Could you check a few things on this model? Use its own coordinates, in mm. A direction names the side the tool comes from. Give positions to 0.01 mm unless a question says otherwise; leave off trailing zeros. Order: outer loops, then holes, each group sorted by start corner. A loop starts at its lowest first (then second) coordinate and runs counter-clockwise, first axis right, second up. Notation, with made-up numbers: (71.5, 86.25) - (93.5, 86.25) arc R36 ccw to (93.5, 120.25) - close; hole circle Ø4 at (31.25, -6). An arc over 180 degrees is marked (long way). One line per question, with ' | ' between items. Start each with the question number.
1. Imagine slicing it at C-C (y = -45). Please give me the cut outline in (x, z), and give its area (3 significant figures).
2. If we mould it in two halves opening along Y, with no side actions, what happens to faces 1 (the cylindrical face through (-0.2, 18.95, -0.22)), 2 (the flat face through (-3, -54.33, 2)), 3 (the cylindrical face through (-3.905, -56.056, 0.867))? For each: released by +Y, released by -Y, zero draft, split by the parting line, or undercut.
3. I need wall thicknesses on probe 1 along X at (y, z) = (-36.5, -5.5); probe 2 along X at (y, z) = (3, 8). Which ranges of each line are inside material? Lowest first, please. Write a range as from..to.
4. For P1, Ø6.5, axis at x = 0.5, z = 1, coming from the +Y side; P2, Ø8, axis at x = 4.5, y = -24.5, coming from the -Z side; P3, Ø12, axis at x = 11.5, z = -13, coming from the -Y side, each with a flat end and sliding along its axis, tell me the tip position at first contact or that it passes through.
5. Which directions (+Z, -Z, +X, -X, +Y, -Y) give clear straight access to the entire face, cutting with the end or side of a thin tool? Please do faces 4 (the flat face through (0, -57.07, 0)), 5 (the cylindrical face through (-1.93, -54.71, 2.52)), 6 (the flat face through (-4.1, -39.57, -1.3)).
6. Imagine slicing it at D-D (y = -7.5). Please give me the cut outline in (x, z), and give its area (3 significant figures).
7. Imagine slicing it at A-A (z = 0). Please give me the cut outline in (x, y) (3 decimals).
8. Imagine slicing it at B-B (x = 0). Please give me the cut outline in (y, z) (3 decimals).
```python
from build123d import *

# Parameters (mm, degrees)
SKETCH1_R               = 16
BOSS_EXTRUDE1_DEPTH     = 24
SKETCH2_R               = 6.35
BOSS_EXTRUDE2_DEPTH     = 39.57
SKETCH3_R               = 4
BOSS_EXTRUDE3_DEPTH     = 17.5
CUT_EXTRUDE1_DEPTH      = 62.392058933
CUT_EXTRUDE1_DEPTH_BACK = 62.392058933
SKETCH4_R               = 19.05
CUT_EXTRUDE2_START      = -2
SKETCH5_R               = 4.571040919
SKETCH5_R_2             = 3.175
CUT_EXTRUDE2_DEPTH      = 0.74


with BuildPart() as part:
    # Sketch1 → Boss-Extrude1 (new body)
    with BuildSketch(Plane(origin=(0, 0, 0), x_dir=(1, 0, 0), z_dir=(0, 1, 0))):
        with Locations(Location((0, 0, 0), (0, 0, 270))):
            Circle(SKETCH1_R)
    extrude(amount=BOSS_EXTRUDE1_DEPTH)

    # Sketch2 → Boss-Extrude2 (add)
    with BuildSketch(Plane.XZ):
        with Locations(Location((0, 0, 0), (0, 0, 270))):
            Circle(SKETCH2_R)
    extrude(amount=BOSS_EXTRUDE2_DEPTH)

    # Sketch3 → Boss-Extrude3 (add)
    with BuildSketch(Plane.XZ.offset(39.57)):
        with Locations(Location((0, 0, 0), (0, 0, 270))):
            Circle(SKETCH3_R)
    extrude(amount=BOSS_EXTRUDE3_DEPTH)

    # Sketch4 → Cut-Extrude1 (cut, two sides: drawn at the far end of the back side and taken through both)
    with BuildSketch(Plane.XY.offset(-CUT_EXTRUDE1_DEPTH_BACK)):
        with Locations((0, 38)):
            Circle(SKETCH4_R)
    extrude(amount=CUT_EXTRUDE1_DEPTH + CUT_EXTRUDE1_DEPTH_BACK, mode=Mode.SUBTRACT)

    # Sketch5 → Cut-Extrude2 (cut)
    with BuildSketch(Plane.XZ.offset(57.07).offset(CUT_EXTRUDE2_START)):
        Circle(SKETCH5_R)
        with Locations(Location((0, 0, 0), (0, 0, 270))):
            Circle(SKETCH5_R_2, mode=Mode.SUBTRACT)
    extrude(amount=-CUT_EXTRUDE2_DEPTH, mode=Mode.SUBTRACT)


solid = part.part
```
Results found:
1) outline: circle Ø8 at (0, 0) | area: 50.3 mm2
2) face 1: released by +Y | face 2: undercut | face 3: zero draft
3) probe 1: x = -3.17..3.17 | probe 2: x = -13.86..13.86
4) P1: stops at y = 19.32 | P2: stops at z = -6.33 | P3: stops at y = 0
5) face 4: +Z, -Z, +X, -X, -Y | face 5: none | face 6: -Y
6) outline: circle Ø12.7 at (0, 0) | area: 127 mm2
7) outline: (-16, 0) - (-6.35, 0) - (-6.35, -39.57) - (-4, -39.57) - (-4, -54.33) - (-3.175, -54.33) - (-3.175, -55.07) - (-4, -55.07) - (-4, -57.07) - (4, -57.07) - (4, -55.07) - (3.175, -55.07) - (3.175, -54.33) - (4, -54.33) - (4, -39.57) - (6.35, -39.57) - (6.35, 0) - (16, 0) - (16, 24) - (12.919, 24) arc R19.05 cw to (-12.919, 24) - (-16, 24) - close
8) outline: (-57.07, -4) - (-55.07, -4) - (-55.07, -3.175) - (-54.33, -3.175) - (-54.33, -4) - (-39.57, -4) - (-39.57, -6.35) - (0, -6.35) - (0, -16) - (18.95, -16) - (18.95, 16) - (0, 16) - (0, 6.35) - (-39.57, 6.35) - (-39.57, 4) - (-54.33, 4) - (-54.33, 3.175) - (-55.07, 3.175) - (-55.07, 4) - (-57.07, 4) - close
